Geometry: final body of the model. Coordinates: model frame, mm. A direction names the side the tool comes from. Round coordinates to 2 decimals unless told otherwise and drop trailing zeros. Loops run counter-clockwise (first coordinate to the right, second up) from the corner with the lowest first, then second, coordinate; pieces in that order, holes last. Notation, with made-up numbers: (10, -12.5) - (59, -12.5) arc R21 cw to (59, 15.5) - close; hole circle Ø11 at (-37, -15). An arc over 180 degrees is marked (long way). Answer as a JSON object with one key per item and string values. Group by question number.
Item 1: Section C-C (y = -26). Return the cut outline in (x, z), plus the area to 3 significant figures.
Item 2: Section B-B (x = 78.5). Return the cut outline in (y, z).
Item 3: Reachability of faces 1 (the face through (60.6, 10.4, -34.5)), 2 (the face through (54.36, -32.61, -19.23)), 3 (the face through (87, 0, -37)) from +Z, -Z, +X, -X, +Y, -Y: full face, straight path, thin tool, end or side. Return the list, or none.
Item 4: Draft query along X for faces 4 (the face through (121.822, 0, -19)), 5 (the face through (86, 0, -39)), 6 (the face through (54.357, 32.462, -19.227)), 7 (the face through (69.822, -1, -35)). Return one class per face: released by +X, released by -X, zero draft, split by the parting line, or undercut.
Item 5: Section A-A (z = -25.5). Return the cut outline in (x, y).
Item 6: Section D-D (y = -3). Return the cut outline in (x, z), plus the area to 3 significant figures.
Item 7: Line query: line 1 (X direction, y = 25.5, z = -31); line 2 (Y direction, x = 82, z = -17); line 3 (Z direction, x = 97.5, y = 24.5). Output: solid intervals per line, ascending.
Item 8: First-contact query: pin 1 (17 mm diameter, centred on x = 95, y = 14.5, fed in from +Z); pin 2 (1.8 mm diameter, centred on x = 60.61, y = -20.63, fed in from +Z). Flat tips, straight axial feed; report the tip coordinate or a pass-through.
```python
from build123d import *

# Parameters (mm, degrees)
SKETCH1_W           = 70
SKETCH1_H           = 70
BOSS_EXTRUDE1_DEPTH = 39
CHAMFER1_SIZE       = 5
SHELL1_T            = -2
SKETCH3_W           = 2.5
SKETCH3_H           = 66
BOSS_EXTRUDE2_DEPTH = 5
SKETCH4_W           = 13.5
SKETCH4_H           = 3
BOSS_EXTRUDE3_DEPTH = 5
SKETCH5_W           = 13.5
SKETCH5_H           = 5.5
CUT_EXTRUDE1_DEPTH  = 133.059792404
SKETCH6_R           = 6.25
CUT_EXTRUDE2_DEPTH  = 133.059792404
CUT_EXTRUDE3_DEPTH  = 10
SKETCH9_R           = 2
BOSS_EXTRUDE4_DEPTH = 5
SKETCH10_R          = 1.1
CUT_EXTRUDE4_DEPTH  = 4


with BuildPart() as part:
    # Sketch1 → Boss-Extrude1 (new body)
    with BuildSketch(Plane.XY):
        with Locations((86.822194683, -0.073375262)):
            Rectangle(SKETCH1_W, SKETCH1_H)
    extrude(amount=-BOSS_EXTRUDE1_DEPTH)

    # Chamfer1
    chamfer1_edges = [part.edges().sort_by_distance(p)[0] for p in [
        (51.822194683, 34.926624738, -19.5),
        (121.822194683, 34.926624738, -19.5),
        (121.822194683, -35.073375262, -19.5),
        (51.822194683, -35.073375262, -19.5),
    ]]
    chamfer(chamfer1_edges, length=CHAMFER1_SIZE)

    # Shell1
    shell1_openings = [part.faces().sort_by_distance(p)[0] for p in [
        (86.822194683, -0.073375262, 0),
    ]]
    offset(amount=SHELL1_T, openings=shell1_openings, kind=Kind.INTERSECTION)

    # Sketch3 → Boss-Extrude2 (add)
    with BuildSketch(Plane.XY.offset(-37)):
        with Locations((68.572194683, -0.073375262)):
            Rectangle(SKETCH3_W, SKETCH3_H)
        with Locations((105.072194683, -0.073375262)):
            Rectangle(SKETCH3_W, SKETCH3_H)
    extrude(amount=BOSS_EXTRUDE2_DEPTH)

    # Sketch4 → Boss-Extrude3 (add)
    with BuildSketch(Plane.XY.offset(-37)):
        with Locations((60.572194683, -20.573375262)):
            Rectangle(SKETCH4_W, SKETCH4_H)
        with Locations((60.572194683, 8.426624738)):
            Rectangle(SKETCH4_W, SKETCH4_H)
        with Locations((113.072194683, -20.573375262)):
            Rectangle(SKETCH4_W, SKETCH4_H)
        with Locations((113.072194683, 8.426624738)):
            Rectangle(SKETCH4_W, SKETCH4_H)
    extrude(amount=BOSS_EXTRUDE3_DEPTH)

    # Sketch5 → Cut-Extrude1 (cut, through all)
    with BuildSketch(Plane.XY.offset(-37)):
        with Locations((60.572194683, 12.676624738)):
            Rectangle(SKETCH5_W, SKETCH5_H)
        with Locations((113.072194683, 12.676624738)):
            Rectangle(SKETCH5_W, SKETCH5_H)
    extrude(amount=-CUT_EXTRUDE1_DEPTH, mode=Mode.SUBTRACT)

    # Sketch6 → Cut-Extrude2 (cut, through all)
    with BuildSketch(Plane.XY.offset(-37)):
        with Locations((60.586585442, -0.573375262)):
            Circle(SKETCH6_R)
        with Locations(Location((113.057803924, -0.573375262, 0), (0, 0, 180))):
            Circle(SKETCH6_R)
    extrude(amount=-CUT_EXTRUDE2_DEPTH, mode=Mode.SUBTRACT)

    # Sketch8 → Cut-Extrude3 (cut)
    with BuildSketch(Plane.XY.offset(-37)):
        with BuildLine():
            Line((58.792309456, -6.560283787), (62.384377825, -6.559228798))
            ThreePointArc((62.384377825, -6.559228798), (60.589297041, -9.805930725), (58.792309456, -6.560283787))
        make_face()
        with BuildLine():
            Line((114.85207991, -6.560283787), (111.260011542, -6.559228798))
            ThreePointArc((111.260011542, -6.559228798), (113.055092325, -9.805930725), (114.85207991, -6.560283787))
        make_face()
    extrude(amount=-CUT_EXTRUDE3_DEPTH, mode=Mode.SUBTRACT)

    # Sketch9 → Boss-Extrude4 (add)
    with BuildSketch(Plane.XY.offset(-32)):
        with Locations((60.59354187, 8.400826661)):
            Circle(SKETCH9_R)
        with Locations((60.59354187, -20.414986166)):
            Circle(SKETCH9_R)
        with Locations((113.050847497, -20.414986166)):
            Circle(SKETCH9_R)
        with Locations((113.050847497, 8.400826661)):
            Circle(SKETCH9_R)
    extrude(amount=-BOSS_EXTRUDE4_DEPTH)

    # Sketch10 → Cut-Extrude4 (cut)
    with BuildSketch(Plane.XY.offset(-32)):
        with Locations((60.60651545, 8.30988812)):
            Circle(SKETCH10_R)
        with Locations((60.60651545, -20.632962205)):
            Circle(SKETCH10_R)
        with Locations(Location((113.037873916, -20.632962205, 0), (0, 0, 180))):
            Circle(SKETCH10_R)
        with Locations(Location((113.037873916, 8.30988812, 0), (0, 0, 180))):
            Circle(SKETCH10_R)
    extrude(amount=-CUT_EXTRUDE4_DEPTH, mode=Mode.SUBTRACT)


solid = part.part
```
Values:
{
 "1": {"outline": "(51.82, -39) - (121.82, -39) - (121.82, 0) - (119.82, 0) - (119.82, -37) - (106.32, -37) - (106.32, -32) - (103.82, -32) - (103.82, -37) - (69.82, -37) - (69.82, -32) - (67.32, -32) - (67.32, -37) - (53.82, -37) - (53.82, 0) - (51.82, 0) - close", "area": "313 mm^2"},
 "2": {"outline": "(-35.07, -39) - (34.93, -39) - (34.93, 0) - (32.93, 0) - (32.93, -37) - (-33.07, -37) - (-33.07, 0) - (-35.07, 0) - close"},
 "3": {"face 1": "+Z, -Z", "face 2": "+Z, -Z, -X, -Y", "face 3": "+Z"},
 "4": {"face 4": "released by +X", "face 5": "zero draft", "face 6": "released by -X", "face 7": "undercut"},
 "5": {"outline": "(51.82, -30.07) - (56.82, -35.07) - (116.82, -35.07) - (121.82, -30.07) - (121.82, 29.93) - (116.82, 34.93) - (56.82, 34.93) - (51.82, 29.93) - close; hole (53.82, -29.24) - (57.65, -33.07) - (115.99, -33.07) - (119.82, -29.24) - (119.82, 29.1) - (115.99, 32.93) - (57.65, 32.93) - (53.82, 29.1) - close"},
 "6": {"outline": "(51.82, -39) - (54.83, -39) - (54.83, -37) - (53.82, -37) - (53.82, 0) - (51.82, 0) - close; (66.35, -39) - (107.3, -39) - (107.3, -37) - (106.32, -37) - (106.32, -32) - (103.82, -32) - (103.82, -37) - (69.82, -37) - (69.82, -32) - (67.32, -32) - (67.32, -37) - (66.35, -37) - close; (118.82, -39) - (121.82, -39) - (121.82, 0) - (119.82, 0) - (119.82, -37) - (118.82, -37) - close", "area": "267 mm^2"},
 "7": {"line 1": "x = 51.82 to 53.82, 119.82 to 121.82", "line 2": "y = -35.07 to -33.07, 32.93 to 34.93", "line 3": "z = -39 to -37"},
 "8": {"pin 1": "stops at z = -37", "pin 2": "stops at z = -36"}
}
